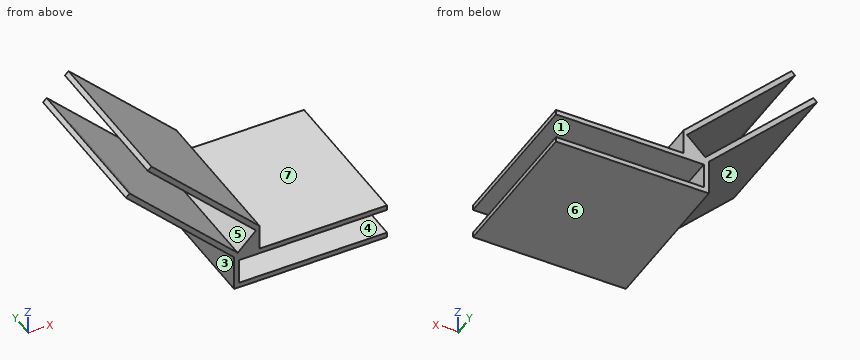
```python
from build123d import *

# Parameters (mm, degrees)
SKETCH1_W           = 30
SKETCH1_H           = 30
BOSS_EXTRUDE1_DEPTH = 7
SHELL1_T            = -1
SKETCH2_W           = 30
SKETCH2_H           = 7
BOSS_EXTRUDE2_DEPTH = 30
SKETCH3_W           = 30
SKETCH3_H           = 7
BOSS_EXTRUDE3_DEPTH = 30
SKETCH5_W           = 5
SKETCH5_H           = 23
BOSS_EXTRUDE4_DEPTH = 5
CUT_EXTRUDE6_DEPTH  = 23
SKETCH12_W          = 7.071067812
SKETCH12_H          = 23
BOSS_EXTRUDE6_DEPTH = 30
CUT_EXTRUDE7_DEPTH  = 22
CUT_EXTRUDE8_DEPTH  = 22
SHELL2_START        = 24
SHELL2_DEPTH        = 5
SHELL2_START_2      = 23
SHELL2_2_DEPTH      = 1
SHELL2_START_3      = 1
SHELL2_3_DEPTH      = 22
BOSS_EXTRUDE7_DEPTH = 1
BOSS_EXTRUDE8_DEPTH = 23
CUT_EXTRUDE10_DEPTH = 1
CUT_EXTRUDE11_DEPTH = 7
BOSS_EXTRUDE9_DEPTH = 7
CUT_EXTRUDE12_DEPTH = 7
SKETCH23_W          = 29
SKETCH23_H          = 5
CUT_EXTRUDE14_DEPTH = 7
CUT_EXTRUDE15_DEPTH = 7


# Read off the part's stored shape, not the designer's step: Shell2
with BuildPart() as part:
    # Sketch1 → Boss-Extrude1 (new body)
    with BuildSketch(Plane.XY):
        with Locations((15, 15)):
            Rectangle(SKETCH1_W, SKETCH1_H)
    extrude(amount=BOSS_EXTRUDE1_DEPTH)

    # Shell1
    shell1_openings = [part.faces().sort_by_distance(p)[0] for p in [
        (30, 15, 3.5),
        (15, 0, 3.5),
    ]]
    offset(amount=SHELL1_T, openings=shell1_openings, kind=Kind.INTERSECTION)

    # Sketch2 → Boss-Extrude2 (add)
    with BuildSketch(Plane.XY.offset(7)):
        with Locations((15, 26.5)):
            Rectangle(SKETCH2_W, SKETCH2_H)
    extrude(amount=BOSS_EXTRUDE2_DEPTH)

    # Sketch3 → Boss-Extrude3 (add)
    with BuildSketch(Plane.ZY):
        with Locations((22, 26.5)):
            Rectangle(SKETCH3_W, SKETCH3_H)
    extrude(amount=BOSS_EXTRUDE3_DEPTH)

    # Sketch5 → Boss-Extrude4 (add)
    with BuildSketch(Plane.XY.offset(7)):
        with Locations((2.5, 11.5)):
            Rectangle(SKETCH5_W, SKETCH5_H)
    extrude(amount=BOSS_EXTRUDE4_DEPTH)

    # Sketch6 → Cut-Extrude6 (cut)
    with BuildSketch(Plane.XZ):
        Polygon((0, 12), (5, 12), (0, 7), align=None)
    extrude(amount=-CUT_EXTRUDE6_DEPTH, mode=Mode.SUBTRACT)

    # Sketch12 → Boss-Extrude6 (add)
    with BuildSketch(Plane(origin=(-3.5, 0, 3.5), x_dir=(0.7071067811865475, 0, 0.7071067811865477), z_dir=(-0.7071067811865477, 0, 0.7071067811865475))):
        with Locations((8.485281374, 11.5)):
            Rectangle(SKETCH12_W, SKETCH12_H)
    extrude(amount=BOSS_EXTRUDE6_DEPTH)

    # Sketch13 → Cut-Extrude7 (cut)
    with BuildSketch(Plane.XZ):
        Polygon((-19.798989873, 28.213203436), (0.707106781, 7.707106781), (4.292893219, 11.292893219), (-16.213203436, 31.798989873), (-16.920310217, 32.506096654), (-20.506096654, 28.920310217), align=None)
    extrude(amount=-CUT_EXTRUDE7_DEPTH, mode=Mode.SUBTRACT)

    # Sketch4 → Cut-Extrude8 (cut)
    with BuildSketch(Plane.XZ.offset(-23)):
        Polygon((-30, 37), (0, 7), (-30, 7), align=None)
    extrude(amount=-CUT_EXTRUDE8_DEPTH, mode=Mode.SUBTRACT)

    # Shell2 outline → Shell2 (cut)
    with BuildSketch(Plane(origin=(0, 0, 0), x_dir=(1, 0, 0), z_dir=(0, 1, 0)).offset(SHELL2_START)):
        Polygon((29, -37), (29, -7), (1, -7), (1, -7.414213562), (-28.585786438, -37), align=None)
    extrude(amount=SHELL2_DEPTH, mode=Mode.SUBTRACT)

    # Shell2 2 outline → Shell2 2 (cut)
    with BuildSketch(Plane(origin=(0, 0, 0), x_dir=(1, 0, 0), z_dir=(0, 1, 0)).offset(SHELL2_START_2)):
        Polygon((4, -7), (1, -7), (1, -7.414213562), (-19.798989873, -28.213203435), (-16.213203436, -31.798989873), (4, -11.585786438), align=None)
    extrude(amount=SHELL2_2_DEPTH, mode=Mode.SUBTRACT)

    # Shell2 3 outline → Shell2 3 (cut)
    with BuildSketch(Plane(origin=(0, 0, 0), x_dir=(1, 0, 0), z_dir=(0, 1, 0)).offset(SHELL2_START_3)):
        Polygon((4, -9.585786438), (4, -7), (1.414213562, -7), align=None)
    extrude(amount=SHELL2_3_DEPTH, mode=Mode.SUBTRACT)

    # Sketch16 → Boss-Extrude7 (add)
    with BuildSketch(Plane(origin=(0, 23, 0), x_dir=(1, 0, 0), z_dir=(0, 1, 0))):
        Polygon((1.414213562, -7), (1, -7), (1, -7.414213562), (-19.798989873, -28.213203436), (-16.213203436, -31.798989873), (4, -11.585786438), (4, -9.585786438), align=None)
    extrude(amount=BOSS_EXTRUDE7_DEPTH)

    # Sketch18 → Boss-Extrude8 (add)
    with BuildSketch(Plane(origin=(0, 1, 0), x_dir=(1, 0, 0), z_dir=(0, 1, 0))):
        Polygon((4, -9.585786438), (4, -7), (1.414213562, -7), align=None)
    extrude(amount=BOSS_EXTRUDE8_DEPTH)

    # Sketch19 → Cut-Extrude10 (cut)
    with BuildSketch(Plane(origin=(30, 0, 0), x_dir=(0, 0, -1), z_dir=(1, 0, 0))):
        Polygon((-36, 29), (-37, 29), (-37, 24), (-36, 24), (-7, 24), (-7, 29), align=None)
    extrude(amount=-CUT_EXTRUDE10_DEPTH, mode=Mode.SUBTRACT)

    # Sketch17 → Cut-Extrude11 (cut)
    with BuildSketch(Plane(origin=(0, 30, 0), x_dir=(1, 0, 0), z_dir=(0, 1, 0))):
        Polygon((0, -7), (30, -7), (30, -37), (-30, -37), align=None)
    extrude(amount=-CUT_EXTRUDE11_DEPTH, mode=Mode.SUBTRACT)

    # Sketch21 → Boss-Extrude9 (add)
    with BuildSketch(Plane(origin=(0, 23, 0), x_dir=(1, 0, 0), z_dir=(0, 1, 0))):
        Polygon((5, -12), (5, -7), (0, -7), (-21.213203436, -28.213203436), (-16.213203436, -33.213203436), align=None)
    extrude(amount=BOSS_EXTRUDE9_DEPTH)

    # Sketch22 → Cut-Extrude12 (cut)
    with BuildSketch(Plane.XZ.offset(-22)):
        Polygon((-16.920310217, 32.506096654), (-20.506096654, 28.920310217), (0.707106781, 7.707106781), (4.292893219, 11.292893219), align=None)
    extrude(amount=-CUT_EXTRUDE12_DEPTH, mode=Mode.SUBTRACT)

    # Sketch23 → Cut-Extrude14 (cut)
    with BuildSketch(Plane(origin=(0, 30, 0), x_dir=(1, 0, 0), z_dir=(0, 1, 0))):
        with Locations((15.5, -3.5)):
            Rectangle(SKETCH23_W, SKETCH23_H)
    extrude(amount=-CUT_EXTRUDE14_DEPTH, mode=Mode.SUBTRACT)

    # Sketch24 → Cut-Extrude15 (cut)
    with BuildSketch(Plane.XZ.offset(-29)):
        Polygon((4.292893219, 11.292893219), (-16.920310217, 32.506096654), (-20.506096654, 28.920310217), (0.707106781, 7.707106781), align=None)
    extrude(amount=-CUT_EXTRUDE15_DEPTH, mode=Mode.SUBTRACT)


solid = part.part
```
Input: part model. Units: mm. Frame: model coordinates. Face numbers are marked on the shaded views. A direction names the side the tool comes from. Give positions to 0.01 mm unless a question says otherwise; leave off trailing zeros. Write each loop counter-clockwise with the first axis right and the second up, starting at its lowest first coordinate (ties: lowest second). Pieces come first, ordered by that corner, then holes. Notation, with made-up numbers: (68, 75) - (78, 75) arc R29 cw to (78, 106) - close; hole circle Ø5 at (78, 58.25). An arc over 180 degrees is marked (long way). Write item = value, one per line. Start each with the question number.
1) Cut plane A-A (x = 24). Return loops of the section in (y, z), and give its area (3 significant figures).
2) Pin query (flat end, axial travel): pin 1 (12 mm diameter, centred on x = 1, z = 13, fed in from +Y); pin 2 (10 mm diameter, centred on x = -13.5, z = 7.5, fed in from +Y) (3 decimals); pin 3 (2 mm diameter, centred on x = 9.5, y = 22, fed in from +Z); pin 4 (1 mm diameter, centred on y = 11, z = 9, fed in from -X). Return the tip coordinate at first contact, or that it passes through.
3) Cut plane C-C (x = 3.5). Return loops of the section in (y, z), and give its area (3 significant figures).
4) Reachability of the marked faces 4, 5, 6 and 7 from +Z, -Z, +X, -X, +Y, -Y: full face, straight path, thin tool, end or side. Return the list, or none.
5) Cut plane D-D (z = 27). Return loops of the section in (x, y), and give its area (3 significant figures).
6) Material intervals for L1, parallel to Z at x = 20.5, y = 14.25; L2, parallel to Z at x = 4.5, y = 12; L3, parallel to X at y = 5.25, z = 25, sorted ascending. Write a range as [from, to].
7) Draft query along Z for the marked faces 1, 2 and 3. Return one class per face: pulls with the +Z half, pulls with the -Z half, needs draft (parallel to the pull), parting line crosses it, or undercut.
8) Cut plane B-B (y = 16.25). Return loops of the section in (x, z), and give its area (4 significant figures).
Answers follow:
q1.outline = (0, 0) - (30, 0) - (30, 1) - (0, 1) - close; (0, 6) - (30, 6) - (30, 7) - (0, 7) - close
q1.area = 60.0 mm^2
q2.pin_1 = 30
q2.pin_2 = through
q2.pin_3 = 7
q2.pin_4 = -2.5
q3.outline = (0, 0) - (30, 0) - (30, 1) - (0, 1) - close; (0, 6) - (30, 6) - (30, 10.5) - (0, 10.5) - close; (0, 12.09) - (30, 12.09) - (30, 13.5) - (0, 13.5) - close
q3.area = 207 mm^2
q4.face_4 = +X, +Y, -Y
q4.face_5 = +Y, -Y
q4.face_6 = -Z, +X, -X, +Y, -Y
q4.face_7 = +Z, +X, +Y, -Y
q5.outline = (-20, 0) - (-18.59, 0) - (-18.59, 30) - (-20, 30) - close; (-11.41, 0) - (-10, 0) - (-10, 30) - (-11.41, 30) - close
q5.area = 84.9 mm^2
q6.L1 = [0, 1], [6, 7]
q6.L2 = [0, 1], [6, 12.5]
q6.L3 = [-18, -16.59], [-9.41, -8]
q7.face_1 = undercut
q7.face_2 = pulls with the -Z half
q7.face_3 = needs draft
q8.outline = (-21.21, 28.21) - (0, 7) - (0, 0) - (30, 0) - (30, 1) - (1, 1) - (1, 6) - (30, 6) - (30, 7) - (5, 7) - (5, 12) - (-16.21, 33.21) - (-16.92, 32.51) - (4.29, 11.29) - (0.71, 7.71) - (-20.51, 28.92) - close
q8.area = 137.5 mm^2
